```python
from build123d import *

# Parameters (mm, degrees)
SKETCH_1_W             = 40
SKETCH_1_H             = 8
EXTRUDE_1_DEPTH        = 4
HOLE_WIZARD_M4_1_D     = 3.3
HOLE_WIZARD_M4_1_DEPTH = 10.1
HOLE_WIZARD_M4_1_TIP   = 0.991420021
HOLE_WIZARD_M4_2_D     = 3.3
HOLE_WIZARD_M4_2_DEPTH = 10.1
HOLE_WIZARD_M4_2_TIP   = 0.991420021
CHAMFER_1_SIZE         = 0.5


with BuildPart() as part:
    # 草图1 → 凸台-拉伸1 (new, symmetric)
    with BuildSketch(Plane.XY):
        Rectangle(SKETCH_1_W, SKETCH_1_H)
    extrude(amount=EXTRUDE_1_DEPTH, both=True)

    # M4 螺纹孔1
    with Locations(Plane.XY.offset(4)):
        with Locations((-15, 0), (15, 0)):
            Hole(HOLE_WIZARD_M4_1_D / 2, depth=HOLE_WIZARD_M4_1_DEPTH)
            with Locations((0, 0, -(HOLE_WIZARD_M4_1_DEPTH + HOLE_WIZARD_M4_1_TIP / 2))):  # 118° drill point
                Cone(0, HOLE_WIZARD_M4_1_D / 2, HOLE_WIZARD_M4_1_TIP, mode=Mode.SUBTRACT)

    # M4 螺纹孔2
    with Locations(Plane(origin=(0, 4, 0), x_dir=(1, 0, 0), z_dir=(0, 1, 0))):
        with Locations((0, 0)):
            Hole(HOLE_WIZARD_M4_2_D / 2, depth=HOLE_WIZARD_M4_2_DEPTH)
            with Locations((0, 0, -(HOLE_WIZARD_M4_2_DEPTH + HOLE_WIZARD_M4_2_TIP / 2))):  # 118° drill point
                Cone(0, HOLE_WIZARD_M4_2_D / 2, HOLE_WIZARD_M4_2_TIP, mode=Mode.SUBTRACT)

    # 倒角1
    chamfer_1_edges = [part.edges().sort_by_distance(p)[0] for p in [
        (-20, 0, 4),
        (16.65, 0, -4),
        (16.65, 0, 4),
        (0, -4, 4),
        (-13.35, 0, -4),
        (-13.35, 0, 4),
        (1.65, -4, 0),
        (1.65, 4, 0),
        (20, 0, 4),
        (0, -4, -4),
        (-20, 0, -4),
        (0, 4, -4),
        (20, 0, -4),
        (20, -4, 0),
        (-20, -4, 0),
        (-20, 4, 0),
        (20, 4, 0),
        (0, 4, 4),
    ]]
    chamfer(chamfer_1_edges, length=CHAMFER_1_SIZE)


solid = part.part
```
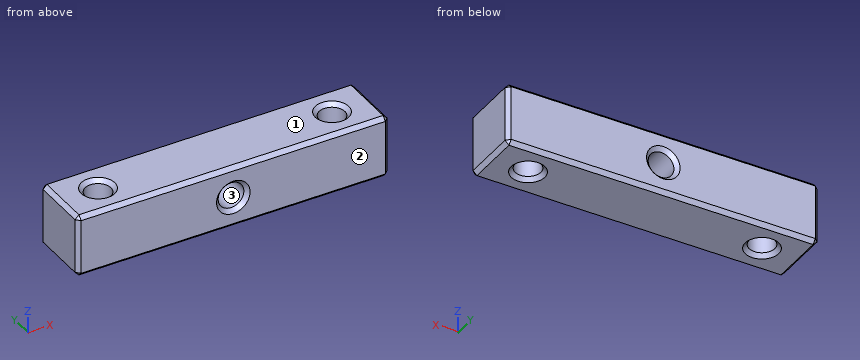
The listing builds one solid part. Answer for the finished solid, in the listing's coordinates (mm). Face numbers are marked on the shaded views. Round coordinates to 2 decimals unless told otherwise and drop trailing zeros. Write each loop counter-clockwise with the first axis right and the second up, starting at its lowest first coordinate (ties: lowest second). Pieces come first, ordered by that corner, then holes. Notation, with made-up numbers: (13, 2.25) -> (20, 2.25) arc R31 ccw to (20, 37.25) -> close; hole circle Ø9 at (9, -7). An arc over 180 degrees is marked (long way). Answer as a JSON object with one key per item and string values. Group by question number.
Q1. Section A-A (z = 0) is taken. Write down the section's boundary in (x, y), plus the area to 3 significant figures.
Q2. Determine the mould class of the marked faces 1, 2 and 3 for opening direction Z: pulls with the +Z half, pulls with the -Z half, needs draft (parallel to the pull), parting line crosses it, or undercut.
Q3. Section D-D (y = 1) is taken. Count the separate pieces of the cut face and the enclosed holes in it, plus the area to 3 significant figures.
Q4. Section C-C (y = 2.5) is taken. Write down the section's boundary in (x, z), plus the area to 3 significant figures.
Q5. Each of these flat-tipped pins is pushed along its axis until it touches: pin 1 Ø4 at (x, y) = (15, 0) entering from +Z; pin 2 Ø3 at (x, z) = (0, 0) entering from +Y; pin 3 Ø4.5 at (x, y) = (-15, 0) entering from -Z. Where does it stop, or does it pass through?
Q6. Section B-B (x = -15) is taken. Write down the section's boundary in (y, z), plus the area to 3 significant figures.
Q7. Straight lines are drawn through the part: line 1 along X through (y, z) = (1.25, 1.5); line 2 along Y through (x, z) = (15, 2); line 3 along X through (y, z) = (1.5, -2.75). For each, find the intervals that lie inside material, in ascending order.
Check values:
{
 "1": {"outline": "(-20, -3.5) -> (-19.5, -4) -> (-2.15, -4) -> (-1.65, -3.5) -> (-1.65, 3.5) -> (-2.15, 4) -> (-19.5, 4) -> (-20, 3.5) -> close; (1.65, -3.5) -> (2.15, -4) -> (19.5, -4) -> (20, -3.5) -> (20, 3.5) -> (19.5, 4) -> (2.15, 4) -> (1.65, 3.5) -> close; hole circle Ø3.3 at (-15, 0); hole circle Ø3.3 at (15, 0)", "area": "275 mm^2"},
 "2": {"face 1": "pulls with the +Z half", "face 2": "needs draft", "face 3": "undercut"},
 "3": {"separate pieces": "3", "enclosed holes": "1", "area": "268 mm^2"},
 "4": {"outline": "(-20, -3.5) -> (-19.5, -4) -> (19.5, -4) -> (20, -3.5) -> (20, 3.5) -> (19.5, 4) -> (-19.5, 4) -> (-20, 3.5) -> close; hole circle Ø3.3 at (0, 0)", "area": "311 mm^2"},
 "5": {"pin 1": "z = 3.85", "pin 2": "through", "pin 3": "z = -4"},
 "6": {"outline": "(-4, -3.5) -> (-3.5, -4) -> (-2.15, -4) -> (-1.65, -3.5) -> (-1.65, 3.5) -> (-2.15, 4) -> (-3.5, 4) -> (-4, 3.5) -> close; (1.65, -3.5) -> (2.15, -4) -> (3.5, -4) -> (4, -3.5) -> (4, 3.5) -> (3.5, 4) -> (2.15, 4) -> (1.65, 3.5) -> close", "area": "36.6 mm^2"},
 "7": {"line 1": "-20 to -16.08, -13.92 to -0.69, 0.69 to 13.92, 16.08 to 20", "line 2": "-4 to -1.65, 1.65 to 4", "line 3": "-20 to -15.69, -14.31 to 14.31, 15.69 to 20"}
}
